Autodesk Fusion 360 part; units mm, degrees
box "长方体基本要素1" add length 28.3 width 27.7 height 24.5 placed x (0, 0, 1) y (1, 0, 0) z (0, 1, 0) at (0, 0, 0)
sketch "草图2" plane through (27.7, 0, 0) normal (1, 0, 0) x (0, 0, -1)
  line L0 (-28.3, 24.5) -> (-28.3, 0)
  line L1 (-28.3, 0) -> (0, 0)
  line L2 (0, 0) -> (0, 24.5)
  line L3 (0, 24.5) -> (-28.3, 24.5)
  line L4 (0, 24.5) -> (4.5, 24.5)
  line L5 (0, 24.5) -> (0, 11.5)
  line L6 (4.5, 24.5) -> (0, 11.5)
  line L7 (4.5, 24.5) -> (2.5, 24.5)
  line L8 (2.5, 24.5) -> (2.5, 40.5)
  line L9 (4.5, 24.5) -> (4.5, 40.5)
  line L10 (2.5, 40.5) -> (4.5, 40.5)
  dimension "d8" = 4.5
  dimension "d9" = 13
  dimension "d10" = 2
  dimension "d11" = 16
extrude "拉伸3" add sketch "草图2" against normal blind 25.2 contours L2 L4 L5 L6 L7 | L4 L7 L8 L9 L10
extrude "拉伸4" cut sketch "草图2" against normal blind 2.5 contours L2 L4 L5 L6 L7 | L4 L7 L8 L9 L10
fillet "圆角4" radius 1 6 edges at (26.45, 24.5, 0) (13.85, 24.5, 28.3) (0, 12.25, 28.3) (0, 24.5, 14.15) (0, 12.25, 0) (1.25, 24.5, 0)
fillet "圆角5" radius 1 5 edges at (27.7, 11.75, 28.3) (27.7, 24.2071, 28.0071) (27.7, 24.5, 14.15) (27.7, 24.2071, 0.2929) (27.7, 11.75, 0)
fillet "圆角6" radius 3 2 edges at (25.2, 40.5, -3.5) (2.5, 40.5, -3.5)
fillet "圆角7" radius 2 1 edges at (13.85, 24.5, -4.5)
sketch "草图3" plane through (0, 0, -2.5) normal (0, 0, 1) x (1, 0, 0)
  arc A0 (5.5, 40.5) -> (2.5, 37.5) centre (5.5, 37.5) ccw
  line L0 (2.5, 37.5) -> (2.5, 24.5)
  line L1 (2.5, 24.5) -> (25.2, 24.5)
  line L2 (25.2, 24.5) -> (25.2, 37.5)
  arc A1 (25.2, 37.5) -> (22.2, 40.5) centre (22.2, 37.5) ccw
  line L3 (22.2, 40.5) -> (5.5, 40.5)
  line L4 (13.85, 40.5) -> (13.85, 37) construction
  line L5 (13.85, 37) -> (13.85, 34.25) construction
  circle A2 centre (13.85, 34.25) radius 2.75
  point P0 (13.85, 40.5)
  dimension "d34" = 3.5
  dimension "d35" = 2.75
  dimension "d36" = 5.5
extrude "拉伸5" cut sketch "草图3" against normal blind 10 contours A2
sketch "草图4" plane through (0, 0, 0) normal (0, -1, 0) x (1, 0, 0)
  arc A0 (27.7, 27.3) -> (26.7, 28.3) centre (26.7, 27.3) ccw
  line L0 (26.7, 28.3) -> (1, 28.3)
  arc A1 (1, 28.3) -> (0, 27.3) centre (1, 27.3) ccw
  line L1 (0, 27.3) -> (0, 1)
  arc A2 (0, 1) -> (1, 0) centre (1, 1) ccw
  line L2 (1, 0) -> (26.7, 0)
  arc A3 (26.7, 0) -> (27.7, 1) centre (26.7, 1) ccw
  line L3 (27.7, 1) -> (27.7, 27.3)
  line L4 (27.7, 28.3) -> (27.7, 0)
  line L5 (8.5, 28.3) -> (8.5, 22.3)
  line L6 (18.7, 28.3) -> (18.7, 22.2)
  line L7 (27.7, 22.2) -> (18.7, 22.2)
  line L8 (0, 11) -> (9.8, 11)
  line L9 (27.7, 11.4) -> (17.7, 11.4)
  line L10 (17.7, 0) -> (17.7, 11.4)
  line L11 (9.8, 0) -> (9.8, 11)
  line L12 (9.8, 22.2) -> (9.8, 22.3)
  line L13 (0, 22.3) -> (8.5, 22.3)
  point P0 (8.5, 28.3)
  point P1 (18.7, 28.3)
  point P2 (0, 22.3)
  point P3 (0, 11)
  point P4 (9.8, 0)
  point P5 (17.7, 0)
  point P6 (27.7, 11.4)
  point P7 (27.7, 22.2)
  dimension "d39" = 8.5
  dimension "d40" = 9
  dimension "d41" = 6
  dimension "d42" = 11
  dimension "d43" = 9.8
  dimension "d44" = 10
  dimension "d45" = 11.4
  dimension "d46" = 6.1
extrude "拉伸6" add sketch "草图4" along normal blind 28 contours L0 L1 L2 L3 L4 L5 L6 L7 L8 L9 L10 L11 L13
extrude "拉伸1" [suppressed]
fillet "圆角1" [suppressed]
fillet "圆角2" [suppressed]
fillet "圆角3" [suppressed]
extrude "拉伸2" [suppressed]
Design review of the part built by this model. Coordinates are the model's own, in mm. A direction names the side the tool comes from. Coordinates: 2 decimals unless noted, no trailing zeros. Order: outer loops, then holes, each group sorted by start corner. A loop starts at its lowest first (then second) coordinate and runs counter-clockwise, first axis right, second up. Notation, with made-up numbers: M 73,-16 L 84,-16 A19 ccw 84,0 Z; hole C -30,10 d7. An arc over 180 degrees is marked long. Use a Markdown table: item, result.
(1) For faces 1 (the flat face through (14, 24.5, 12)), 2 (the flat face through (18.7, -14, 25)), 3 (the flat face through (17.7, -14, 6)), list the 3-axis set-ups (+Z, -Z, +X, -X, +Y, -Y) from which the entire face can be reached by the end or side of a thin tool; tool diameter is ignored.
Worked answers:
| item | result |
|---|---|
| face 1 | +Z, +X, -X, +Y |
| face 2 | +Z, +X, -Y |
| face 3 | -Z, +X, -Y |
(2) For P1, Ø10, axis at x = 18, y = -10.5, coming from the -Z side; P2, Ø3, axis at x = 4, z = 26.5, coming from the -Y side; P3, Ø2.5, axis at x = 24.5, y = -17.5, coming from the +Z side; P4, Ø5, axis at x = 13.85, y = 34.25, coming from the +Z side, all flat-tipped, find the tip position at first contact; note any pin that passes through.
Worked answers:
| item | result |
|---|---|
| P1 | stops at z = 0 |
| P2 | stops at y = 0 |
| P3 | stops at z = 22.2 |
| P4 | passes through |
(3) Add section D-D (y = -6.5). Give the boundary of the cut face in (x, z).
Worked answers:
| item | result |
|---|---|
| outline | M 0,11 L 9.8,11 L 9.8,0 L 17.7,0 L 17.7,11.4 L 27.7,11.4 L 27.7,22.2 L 18.7,22.2 L 18.7,28.3 L 8.5,28.3 L 8.5,22.3 L 0,22.3 Z |
(4) Add section C-C (z = 13.5). Give the boundary of the cut face in (x, y).
Worked answers:
| item | result |
|---|---|
| outline | M 0,-28 L 27.7,-28 L 27.7,23.5 A1 ccw 26.7,24.5 L 1,24.5 A1 ccw 0,23.5 Z |
(5) Wall thickness on probe 1 along Z at (x, y) = (12.5, 28); probe 2 along X at (y, z) = (34, -3); probe 3 along Z at (x, y) = (22.25, 9): over which ranges is each line inside the solid? List them lowest first.
Worked answers:
| item | result |
|---|---|
| probe 1 | z = -4.5 to -2.5 |
| probe 2 | x = 2.5 to 11.11, 16.59 to 25.2 |
| probe 3 | z = 0 to 28.3 |
(6) Add section B-B (x = 13.85). Give the boundary of the cut face in (y, z).
Worked answers:
| item | result |
|---|---|
| outline | M -28,0 L 11.5,0 L 24.18,-4.39 A2 ccw 24.84,-4.5 L 31.5,-4.5 L 31.5,-2.5 L 24.5,-2.5 L 24.5,27.3 A1 ccw 23.5,28.3 L -28,28.3 Z; M 37,-4.5 L 40.5,-4.5 L 40.5,-2.5 L 37,-2.5 Z |
(7) Add section A-A (y = 34.25). Give the boundary of the cut face in (x, z), then the cut area to 3 significant figures.
Worked answers:
| item | result |
|---|---|
| outline | M 2.5,-4.5 L 11.1,-4.5 L 11.1,-2.5 L 2.5,-2.5 Z; M 16.6,-4.5 L 25.2,-4.5 L 25.2,-2.5 L 16.6,-2.5 Z |
| area | 34.4 mm2 |
